Autodesk Inventor part; units mm, degrees
ref_plane "YZ Plane" through (0, 0, 0) normal (1, 0, 0) x (0, 1, 0)
ref_plane "XZ Plane" through (0, 0, 0) normal (0, 1, 0) x (-1, 0, 0)
ref_plane "XY Plane" through (0, 0, 0) normal (0, 0, 1) x (1, 0, 0)
sketch "Sketch1" plane through (0, 0, 0) normal (0, 1, 0) x (-1, 0, 0)
  line L0 (0, 0) -> (89.1742, 0)
  line L1 (29, 31) -> (29, 45)
  line L2 (29, 45) -> (35, 45)
  line L3 (35, 45) -> (35, 25)
  line L4 (14, 17.5) -> (0, 17.5)
  line L5 (0, 12.5) -> (23, 12.5)
  line L6 (19, 20.5) -> (19, 31)
  line L7 (19, 31) -> (29, 31)
  line L8 (35, 25) -> (23, 25)
  line L9 (23, 25) -> (23, 12.5)
  line L10 (0, 17.5) -> (0, 12.5)
  line L11 (19, 20.5) -> (14, 20.5)
  line L12 (14, 20.5) -> (14, 17.5)
  line L13 (35, 25) -> (40, 25)
  line L14 (40, 25) -> (40, 29)
  line L15 (40, 29) -> (35, 29)
  dimension "d3" = 50
  dimension "d4" = 35
  dimension "d5" = 5
  dimension "d6" = 12
  dimension "d7" = 6
  dimension "d8" = 4
  dimension "d9" = 35
  dimension "d10" = 6
  dimension "d11" = 20
  dimension "d12" = 6
  dimension "d14" = 5
  dimension "d15" = 3
  dimension "d22" = 4
  dimension "d23" = 5
revolve "Revolution1" add sketch "Sketch1" angle 360 about axis through (0, 0, 0) along (-1, 0, 0)
chamfer "Chamfer2" distance 1 angle 45 3 edges at (-29, 0, -45) (-19, 0, -31) (0, 0, -17.5)
properties part number "2 nd output shaft" material "Steel, Mild"
CAD build for the part. Positions are in the model's coordinates, mm. A direction names the side the tool comes from. Coordinates: 2 decimals unless noted, no trailing zeros. Loops run counter-clockwise (first coordinate to the right, second up) from the corner with the lowest first, then second, coordinate; pieces in that order, holes last. Notation, with made-up numbers: (73, 54) - (131, 54) arc R21 cw to (131, 68) - close; hole circle Ø8 at (67.25, 33). An arc over 180 degrees is marked (long way). Use one line per item in the form item = value. Start each with the question number.
1) Band-saw the part on C-C (x = -4). Give the cut face in (y, z).
2) Flat gauge pins, fed straight in: pin 1 (3 mm diameter, centred on x = -31, z = -2, fed in from +Y); pin 2 (12 mm diameter, centred on y = -33.5, z = 12.5, fed in from -X); pin 3 (3 mm diameter, centred on x = -29.5, z = -30, fed in from -Y). Where does each tip first touch, or does it go through?
3) Band-saw the part on D-D (x = -15.5). Give the cut face in (y, z), and give its area (3 significant figures).
4) Drill centre lines: L1, parallel to Y at x = -34.75, z = 0; L2, parallel to Y at x = -8, z = 0; L3, parallel to X at y = -24, z = 9.5. Where is each one in solid material? Low to high. Write a range as from..to.
5) Tool access for faces 5 (the face through (-37.47, 25.73, 13.38)), 6 (the face through (-19, -6, 20)), 7 (the face through (0, 3.7, -12.3)): list every direction of +Z, -Z, +X, -X, +Y, -Y with a clear straight run to the whole face (end or side of a thin tool).
6) Two-plate mould, pull along Y, no slides. Class faces 1 (the face through (-23, 11.5, -5.9)), 2 (the face through (-7.409, 10.648, -13.887)), 3 (the face through (-14, 9.2, 15.1)), 4 (the face through (-11.661, 3.755, 11.923)): +Y half, -Y half, draft (parallel to the pull), parting line (faces both ways), or undercut.
Check values:
q1.outline = circle Ø35 at (0, 0); hole circle Ø25 at (0, 0)
q2.pin_1 = 45
q2.pin_2 = -35
q2.pin_3 = -34.75
q3.outline = circle Ø41 at (0, 0); hole circle Ø25 at (0, 0)
q3.area = 829 mm2
q4.L1 = -45..-25, 25..45
q4.L2 = -17.5..-12.5, 12.5..17.5
q4.L3 = -40..-19
q5.face_5 = -X
q5.face_6 = +X
q5.face_7 = +Z, -Z, +X, +Y, -Y
q6.face_1 = undercut
q6.face_2 = parting line
q6.face_3 = draft
q6.face_4 = undercut
